from build123d import *

# Parameters (mm, degrees)
BOSS_EXTRUDE1_DEPTH = 609.6
SKETCH3_W           = 1059.2
SKETCH3_H           = 25.4
CUT_EXTRUDE2_DEPTH  = 30.48


with BuildPart() as part:
    # Sketch2 → Boss-Extrude1 (new, symmetric)
    with BuildSketch(Plane.XY):
        with BuildLine():
            Line((-12.7, -12.7), (12.7, -12.7))
            Line((12.7, -12.7), (12.7, 12.7))
            Line((12.7, 12.7), (11.1125, 12.7))
            ThreePointArc((11.1125, 12.7), (9.989967985, 12.235032015), (9.525, 11.1125))
            Line((9.525, 11.1125), (9.525, -6.35))
            ThreePointArc((9.525, -6.35), (8.59506403, -8.59506403), (6.35, -9.525))
            Line((6.35, -9.525), (-11.1125, -9.525))
            ThreePointArc((-11.1125, -9.525), (-12.235032015, -9.989967985), (-12.7, -11.1125))
            Line((-12.7, -11.1125), (-12.7, -12.7))
        make_face()
    extrude(amount=BOSS_EXTRUDE1_DEPTH, both=True)

    # Sketch3 → Cut-Extrude2 (cut)
    with BuildSketch(Plane(origin=(12.7, 0, 0), x_dir=(0, 0, -1), z_dir=(1, 0, 0))):
        with Locations((80, 0)):
            Rectangle(SKETCH3_W, SKETCH3_H)
    extrude(amount=-CUT_EXTRUDE2_DEPTH, mode=Mode.SUBTRACT)


solid = part.part
Input: part model. Units: mm. Frame: model coordinates. A direction names the side the tool comes from. Coordinates: 2 decimals unless noted, no trailing zeros. Order: outer loops, then holes, each group sorted by start corner. A loop starts at its lowest first (then second) coordinate and runs counter-clockwise, first axis right, second up. Notation, with made-up numbers: M 50,1.5 L 94,1.5 A28 ccw 94,30.5 Z; hole C 27,-37.75 d10. An arc over 180 degrees is marked long. Answer in a Markdown table with one row per item.
(1) Contact query for flat-ended pins moving along their axis: pin 1 Ø1 at (y, z) = (-2, 505.5) entering from -X (3 decimals); pin 2 Ø5 at (x, y) = (6.5, -3) entering from +Z; pin 3 Ø1 at (x, z) = (7, 489) entering from +Y; pin 4 Ø10 at (y, z) = (-6.5, 499.5) entering from -X. Output: stop coordinate, or through.
Numbers:
| item | result |
|---|---|
| pin 1 | stops at x = 9.525 |
| pin 2 | passes through |
| pin 3 | stops at y = -9.31 |
| pin 4 | stops at x = -12.7 |
(2) Material intervals for line 1 (Y direction, x = -7.5, z = 500.5) (3 decimals); line 2 (X direction, y = 8, z = 571.5) (3 decimals); line 3 (X direction, y = -8, z = 519), sorted ascending. Write a range as [from, to].
Numbers:
| item | result |
|---|---|
| line 1 | y = [-12.7, -9.525] |
| line 2 | x = [9.525, 12.7] |
| line 3 | x = [9.06, 12.7] |
(3) Section query B-B, the plane x = -8.5. Output: boundary loops of the cut face in (y, z) (3 decimals).
Numbers:
| item | result |
|---|---|
| outline | M -12.7,449.6 L -9.525,449.6 L -9.525,609.6 L -12.7,609.6 Z |
(4) Access query for faces 1 (the flat face through (9.525, 3, 531)), 2 (the flat face through (0, -12.7, 531)). Directions: +Z, -Z, +X, -X, +Y, -Y. A direction counts if a zero-diameter tool reaches every point of the face in a straight line with its end or side. Return the directions, or none.
Numbers:
| item | result |
|---|---|
| face 1 | +Z, -Z, -X, +Y |
| face 2 | +Z, -Z, +X, -X, -Y |
(5) Section query C-C, the plane y = -1.5. Output: boundary loops of the cut face in (x, z) (3 decimals), plus the area to 3 significant figures.
Numbers:
| item | result |
|---|---|
| outline | M 9.525,449.6 L 12.7,449.6 L 12.7,609.6 L 9.525,609.6 Z |
| area | 508 mm^2 |
